Source: CAD feature listing. Evaluate the final solid. Frame: model axes, mm. Face numbers are marked on the shaded views. A direction names the side the tool comes from. Give positions to 0.01 mm unless a question says otherwise; leave off trailing zeros. Loops run counter-clockwise (first coordinate to the right, second up) from the corner with the lowest first, then second, coordinate; pieces in that order, holes last. Notation, with made-up numbers: (70, 11) - (94, 11) arc R9 ccw to (94, 24) - close; hole circle Ø4 at (48, -40). An arc over 180 degrees is marked (long way). Put each result on its own line as item: value.
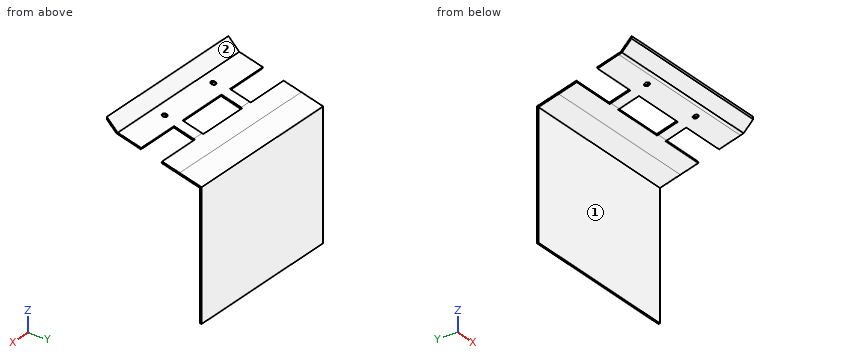
```python
from build123d import *

# Parameters (mm, degrees)
RESSALTO_EXTRUS_O1_DEPTH = 100
RESSALTO_EXTRUS_O2_DEPTH = 100
CORTE_EXTRUS_O1_DEPTH    = 100
RESSALTO_EXTRUS_O3_DEPTH = 100
ESBO_O20_R               = 1.5
CORTE_EXTRUS_O6_DEPTH    = 5
ESBO_O24_W               = 27
ESBO_O24_H               = 13.16698281
ESBO_O24_W_2             = 32
CORTE_EXTRUS_O7_DEPTH    = 115.152987189
CORTE_EXTRUS_O8_DEPTH    = 115.291627571
RESSALTO_EXTRUS_O4_DEPTH = 100


with BuildPart() as part:
    # Esboço1 → Ressalto-extrusão1 (new body)
    with BuildSketch(Plane(origin=(0, 0, 0), x_dir=(0, 0, -1), z_dir=(1, 0, 0))):
        Polygon((0, 0), (9.292893219, 9.292893219), (15.968885233, 32.111148665), (16.934326675, 31.850528592), (10, 8.585786438), (1.414213562, 0), align=None)
    extrude(amount=RESSALTO_EXTRUS_O1_DEPTH)

    # Esboço2 → Ressalto-extrusão2 (add)
    with BuildSketch(Plane(origin=(100, 0, 0), x_dir=(0, 0, -1), z_dir=(1, 0, 0))):
        Polygon((7.816147842, 7.816147842), (14.517472223, 32.825830908), (13.549802648, 33.078052229), (6.665390157, 6.665390157), align=None)
    extrude(amount=-RESSALTO_EXTRUS_O2_DEPTH)

    # Esboço3 → Corte-extrusão1 (cut)
    with BuildSketch(Plane(origin=(100, 0, 0), x_dir=(0, 0, -1), z_dir=(1, 0, 0))):
        Polygon((7.298509752, 5.88429619), (7.816147842, 7.816147842), (9.292893219, 9.292893219), (15.968885233, 32.111148665), (16.934326675, 31.850528592), (10, 8.585786438), align=None)
    extrude(amount=-CORTE_EXTRUS_O1_DEPTH, mode=Mode.SUBTRACT)

    # Esboço4 → Ressalto-extrusão3 (add)
    with BuildSketch(Plane(origin=(100, 0, 0), x_dir=(0, 0, -1), z_dir=(1, 0, 0))):
        Polygon((13.549802648, 33.078052229), (14.517472223, 32.825830908), (19.404372889, 51.574860843), (18.436703315, 51.827082163), align=None)
    extrude(amount=-RESSALTO_EXTRUS_O3_DEPTH)

    # Esboço20 → Corte-extrusão6 (cut)
    with BuildSketch(Plane(origin=(0, -1.202778341, -4.614566301), x_dir=(1, 0, 0), z_dir=(0, 0.25222132052248, 0.9676695745314599))):
        with Locations(Location((30, 14.801620202, 0), (0, 0, 270))):
            Circle(ESBO_O20_R)
        with Locations(Location((70, 14.801620202, 0), (0, 0, 270))):
            Circle(ESBO_O20_R)
    extrude(amount=-CORTE_EXTRUS_O6_DEPTH, mode=Mode.SUBTRACT)

    # Esboço24 → Corte-extrusão7 (cut, through all)
    with BuildSketch(Plane(origin=(0, -1.202778341, -4.614566301), x_dir=(1, 0, 0), z_dir=(0, 0.25222132052248, 0.9676695745314599))):
        with Locations((13.5, 29.585111607)):
            Rectangle(ESBO_O24_W, ESBO_O24_H)
        with Locations((86.5, 29.585111607)):
            Rectangle(ESBO_O24_W, ESBO_O24_H)
        with Locations((50, 29.585111607)):
            Rectangle(ESBO_O24_W_2, ESBO_O24_H)
    extrude(amount=-CORTE_EXTRUS_O7_DEPTH, mode=Mode.SUBTRACT)

    # Esboço25 → Corte-extrusão8 (cut, through all)
    with BuildSketch(Plane(origin=(100, 0, 0), x_dir=(0, 0, -1), z_dir=(1, 0, 0))):
        Polygon((17.579835578, 44.574860843), (10.547206245, 44.574860843), (18.436703315, 51.827082163), (19.404372889, 51.574860843), align=None)
    extrude(amount=-CORTE_EXTRUS_O8_DEPTH, mode=Mode.SUBTRACT)

    # Esboço26 → Ressalto-extrusão4 (add)
    with BuildSketch(Plane(origin=(100, 0, 0), x_dir=(0, 0, -1), z_dir=(1, 0, 0))):
        Polygon((16.546424974, 44.574860843), (17.579835578, 44.574860843), (20.818425576, 57), (63.298509752, 57), (97.298509752, 57), (97.298509752, 58), (63.298509752, 58), (20.045663159, 58), align=None)
    extrude(amount=-RESSALTO_EXTRUS_O4_DEPTH)


solid = part.part
```
1) Section query A-A, the plane x = 7. Output: boundary loops of the cut face in (y, z), plus the area to 3 significant figures.
Check result:
outline: (0, -1.41) - (5.88, -7.3) - (20.82, -11.3) - (21.06, -10.42) - (6.67, -6.67) - (0, 0) - close; (33.54, -14.7) - (57, -20.82) - (57, -97.3) - (58, -97.3) - (58, -20.05) - (33.8, -13.74) - close
area: 123 mm²
2) Section query B-B, the plane y = 23. Output: boundary loops of the cut face in (x, z), plus the area to 3 significant figures.
Check result:
outline: (27, -11.88) - (34, -11.88) - (34, -10.92) - (27, -10.92) - close; (66, -11.88) - (73, -11.88) - (73, -10.92) - (66, -10.92) - close
area: 13.5 mm²
3) Pin query (flat end, axial travel): P1, Ø12, axis at x = 90, y = 39.5, coming from the -Z side; P2, Ø2, axis at x = 27.5, y = 28.5, coming from the +Z side; P3, Ø3.5, axis at y = 27, z = -12.5, coming from the +X side. Return the tip coordinate at first contact, or that it passes through.
Check result:
P1: z = -17.82
P2: z = -12.1
P3: x = 73
4) Access query for the marked faces 1 and 2. Directions: +Z, -Z, +X, -X, +Y, -Y. A direction counts if a zero-diameter tool reaches every point of the face in a straight line with its end or side. Return the directions, or none.
Check result:
face 1: -Z, +X, -X, -Y
face 2: +Z, +X, -X, +Y
5) Section query C-C, the plane z = -40. Output: boundary loops of the cut face in (x, y).
Check result:
outline: (0, 57) - (100, 57) - (100, 58) - (0, 58) - close
6) Material intervals for line 1 along Y through (x, z) = (55.5, -89); line 2 along Z through (x, y) = (40, 34.5); line 3 along Z through (x, y) = (70, 24.5), sorted ascending. Write a range as [from, to].
Check result:
line 1: [57, 58]
line 2: [-14.95, -13.92]
line 3: [-12.29, -11.31]
7) Section query D-D, the plane y = 52.5. Output: boundary loops of the cut face in (x, z).
Check result:
outline: (0, -19.65) - (100, -19.65) - (100, -18.61) - (0, -18.61) - close
